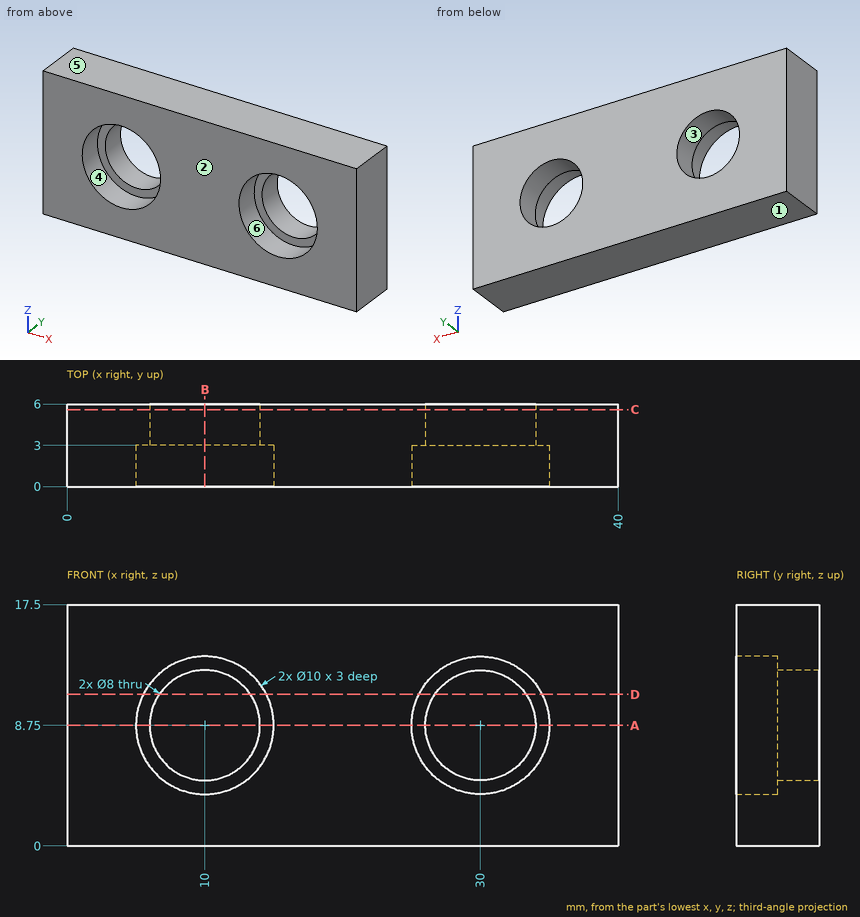
Input: dimensioned drawing with shaded views. Units: mm. Origin: part minimum x, y, z. A direction names the side the tool comes from. Round coordinates to 2 decimals unless told otherwise and drop trailing zeros. Loops run counter-clockwise (first coordinate to the right, second up) from the corner with the lowest first, then second, coordinate; pieces in that order, holes last. Notation, with made-up numbers: M -18.75,5.25 L -7.75,5.25 A17 ccw -7.75,18.25 Z; hole C -4.75,23.5 d5. An arc over 180 degrees is marked long. Return JSON: item names as keys, results as strings. Group by question number.
1. Section query B-B on x = 10. Output: boundary loops of the cut face in (y, z), and give its area (3 significant figures).
2. Pin query (flat end, axial travel): pin 1 (5 mm diameter, centred on x = 31, z = 10, fed in from -Y); pin 2 (7 mm diameter, centred on x = 10, z = 8.75, fed in from -Y). Return the tip coordinate at first contact, or that it passes through.
3. Section query A-A on z = 8.75. Output: boundary loops of the cut face in (x, y).
4. Mould query, pull axis Z, two halves, no side actions, for the marked faces 1, 2, 3 and 4. Classes: released by +Z, released by -Z, zero draft, split by the parting line, or undercut.
5. Section query C-C on y = 5.6. Output: boundary loops of the cut face in (x, z).
6. Material intervals for line 1 along X through (y, z) = (0.9, 8.75); line 2 along Z through (x, y) = (30, 4.3); line 3 along X through (y, z) = (3.9, 8.75), sorted ascending. Write a range as from..to.
7. Reachability of the marked faces 5 and 6 from +Z, -Z, +X, -X, +Y, -Y: full face, straight path, thin tool, end or side. Return the list, or none.
8. Section query D-D on z = 11. Output: boundary loops of the cut face in (x, y).
Checks:
{
 "1": {"outline": "M 0,0 L 6,0 L 6,4.75 L 3,4.75 L 3,3.75 L 0,3.75 Z; M 0,13.75 L 3,13.75 L 3,12.75 L 6,12.75 L 6,17.5 L 0,17.5 Z", "area": "51.0 mm²"},
 "2": {"pin 1": "stops at y = 3", "pin 2": "passes through"},
 "3": {"outline": "M 0,0 L 5,0 L 5,3 L 6,3 L 6,6 L 0,6 Z; M 14,3 L 15,3 L 15,0 L 25,0 L 25,3 L 26,3 L 26,6 L 14,6 Z; M 34,3 L 35,3 L 35,0 L 40,0 L 40,6 L 34,6 Z"},
 "4": {"face 1": "released by -Z", "face 2": "zero draft", "face 3": "undercut", "face 4": "undercut"},
 "5": {"outline": "M 0,0 L 40,0 L 40,17.5 L 0,17.5 Z; hole C 10,8.75 d8; hole C 30,8.75 d8"},
 "6": {"line 1": "x = 0..5, 15..25, 35..40", "line 2": "z = 0..4.75, 12.75..17.5", "line 3": "x = 0..6, 14..26, 34..40"},
 "7": {"face 5": "+Z, +X, -X, +Y, -Y", "face 6": "-Y"},
 "8": {"outline": "M 0,0 L 5.53,0 L 5.53,3 L 6.69,3 L 6.69,6 L 0,6 Z; M 13.31,3 L 14.47,3 L 14.47,0 L 25.53,0 L 25.53,3 L 26.69,3 L 26.69,6 L 13.31,6 Z; M 33.31,3 L 34.47,3 L 34.47,0 L 40,0 L 40,6 L 33.31,6 Z"}
}
